Solid Edge part; units mm, degrees
sketch "Sketch1" plane through (0, 0, 0) normal (0, -1, 0) x (1, 0, 0)
  line L0 (-22.5, -72.5) -> (22.5, -72.5)
  line L1 (22.5, -72.5) -> (22.5, 72.5)
  line L2 (22.5, 72.5) -> (-22.5, 72.5)
  line L3 (-22.5, 72.5) -> (-22.5, -72.5)
extrude "Protrusion1" add sketch "Sketch1" against normal blind 2200
sketch "Sketch2" plane through (-22.5, 1172.7247, 0) normal (-1, 0, 0) x (0, 1, 0)
  line L0 (-1002.2628, 72.5) -> (-933.2816, 60.6007)
  line L1 (-933.2816, 60.6007) -> (-929.9001, 80.2034)
  line L2 (-929.9001, 80.2034) -> (-998.4381, 94.6725)
  line L3 (-998.4381, 94.6725) -> (-1002.2628, 72.5)
extrude "ExtrudedCutout_2" cut sketch "Sketch2" against normal blind 199.504
sketch "Sketch3" plane through (0, 0, 0) normal (0, -1, 0) x (1, 0, 0)
  line L0 (-22.5, -72.5) -> (22.5, -72.5)
  line L1 (22.5, -72.5) -> (22.5, 72.5)
  line L2 (22.5, 72.5) -> (-22.5, 72.5)
  line L3 (-22.5, 72.5) -> (-22.5, -72.5)
extrude "ExtrudedProtrusion_2" add sketch "Sketch3" along normal blind 229.54
sketch "Sketch4" plane through (0, 2200, 22.8323) normal (0, 1, 0) x (-1, 0, 0)
  line L0 (-22.5, -95.3323) -> (22.5, -95.3323)
  line L1 (22.5, -95.3323) -> (22.5, 49.6677)
  line L2 (22.5, 49.6677) -> (-22.5, 49.6677)
  line L3 (-22.5, 49.6677) -> (-22.5, -95.3323)
extrude "ExtrudedProtrusion_3" add sketch "Sketch4" along normal blind 370.46
sketch "Sketch5" plane through (-22.5, 1185.23, 0) normal (-1, 0, 0) x (0, -1, 0)
  line L0 (-1014.77, -72.5) -> (-750.0476, -72.5)
  line L1 (-750.0476, -72.5) -> (-1007.1205, -28.1549)
  line L2 (-1007.1205, -28.1549) -> (-1014.77, -72.5)
extrude "ExtrudedCutout_5" cut sketch "Sketch5" against normal blind 98.6618
properties material "Wood, Pine"
Verification items for the finished model (mm, model axes). A direction names the side the tool comes from. Round coordinates to 2 decimals unless told otherwise and drop trailing zeros. Loops run counter-clockwise (first coordinate to the right, second up) from the corner with the lowest first, then second, coordinate; pieces in that order, holes last. Notation, with made-up numbers: (18, -34) - (53, -34) arc R9 cw to (53, -17) - close; hole circle Ø2 at (17, 1.25). An arc over 180 degrees is marked (long way). Write item = value, one per line.
Q1. Tool access check on faces 1 (the flat face through (0, 1077, -72.5)), 2 (the flat face through (-0.32, 2062.01, -50.64)). Record the directions out of +Z, -Z, +X, -X, +Y, -Y that give a thin tool (end or side, any length) a straight path to the whole face; none if there is none.
Here are the results:
face_1 = -Z, +X, -X, +Y, -Y
face_2 = -Z, +X, -X
Q2. Sectioned sample at A-A on x = -7. Record the boundary of the cut face in (y, z).
Here are the results:
outline = (-229.54, -72.5) - (170.46, -72.5) - (239.44, -60.6) - (241.5, -72.5) - (1935.28, -72.5) - (2192.35, -28.15) - (2200, -72.5) - (2570.46, -72.5) - (2570.46, 72.5) - (-229.54, 72.5) - close
Q3. Sectioned sample at B-B on y = 2154.5. Record the boundary of the cut face in (x, z), plus the area to 3 significant figures.
Here are the results:
outline = (-22.5, -34.68) - (22.5, -34.68) - (22.5, 72.5) - (-22.5, 72.5) - close
area = 4,820 mm^2
Q4. Mould release check, pull along Y, two halves, no side actions. Record for faces 3 (the flat face through (-0.315, 2196.122, -50.017)), 4 (the flat face through (0, -229.54, 1)), 5 (the flat face through (-22.5, 1151, 1)): +Y half, -Y half, draft (parallel to the pull), parting line (faces both ways), or undercut.
Here are the results:
face_3 = undercut
face_4 = -Y half
face_5 = draft
